from build123d import *

# Parameters (mm, degrees)
F0_W     = 127
F0_H     = 76.2
F1_DEPTH = 13.97
F3_D     = 12.7
F4_W     = 12.7
F4_H     = 25.4
F6_W     = 19.05
F6_H     = 12.372993
F8_W     = 9.582032
F8_H     = 12.456644
F10_R    = 2.54
F11_SIZE = 2.54
F12_SIZE = 2.54


with BuildPart() as f1:
    # F0 (on Top) → F1 (new body)
    with BuildSketch(Plane.XY):
        Rectangle(F0_W, F0_H)
    extrude(amount=F1_DEPTH)

    # F3 (through all)
    with Locations(Plane.XY.offset(13.97)):
        with Locations((-44.45, 26.67), (-44.45, -26.67), (44.45, 26.67), (44.45, -26.67)):
            Hole(F3_D / 2)

    # F4 (on Front) → F5 (revolve)
    with BuildSketch(Plane.XZ):
        with Locations((6.35, 26.67)):
            Rectangle(F4_W, F4_H)
    revolve(axis=Axis((0, 0, 26.67), (0, 0, -1)))

    # F6 (on Front) → F7 (revolve)
    with BuildSketch(Plane.XZ):
        with Locations((9.525, 45.556496)):
            Rectangle(F6_W, F6_H)
    revolve(axis=Axis((0, 0, 45.556497), (0, 0, -1)))

    # F8 (on Front) → F9 (revolve)
    with BuildSketch(Plane.XZ):
        with Locations((12.456648, 20.198322)):
            Rectangle(F8_W, F8_H)
    revolve(axis=Axis((0, 0, 13.97), (0, 0, 1)))

    # F10
    f10_edges = [f1.edges().sort_by_distance(p)[0] for p in [
        (-17.247664, 0, 26.426644),
        (-17.247664, 0, 13.97),
        (17.247664, 0, 20.198322),
    ]]
    fillet(f10_edges, radius=F10_R)

    # F11
    f11_edges = [f1.edges().sort_by_distance(p)[0] for p in [
        (-19.05, 0, 51.742993),
    ]]
    chamfer(f11_edges, length=F11_SIZE)

    # F12
    f12_edges = [f1.edges().sort_by_distance(p)[0] for p in [
        (0, -38.1, 13.97),
        (-63.5, 0, 13.97),
        (0, 38.1, 13.97),
        (63.5, 0, 13.97),
    ]]
    chamfer(f12_edges, length=F12_SIZE)


solid = f1.part
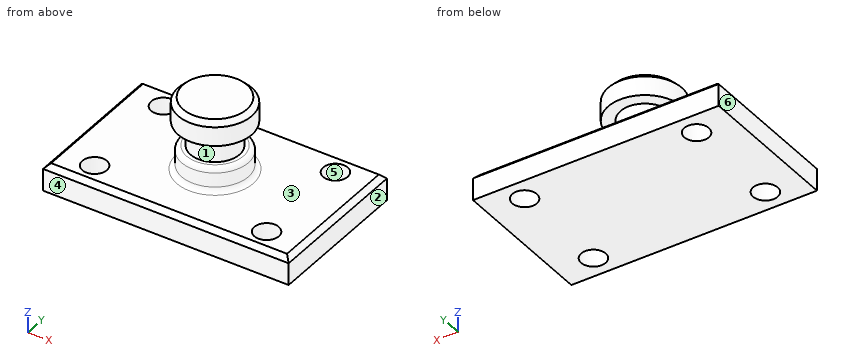
Model file for the job. Use its own axes, mm. Face numbers are marked on the shaded views. A direction names the side the tool comes from. Coordinates: 2 decimals unless noted, no trailing zeros. Write each loop counter-clockwise with the first axis right and the second up, starting at its lowest first coordinate (ties: lowest second). Pieces come first, ordered by that corner, then holes. Notation, with made-up numbers: (-32.5, 13.5) - (4.5, 13.5) arc R27 cw to (4.5, 35.5) - close; hole circle Ø3 at (31, 29). An arc over 180 degrees is marked (long way). Write each question's results on one line, items separated by ' | '. Start each with the question number.
1) 3-axis set-ups, long thin cutter, end or side, ignore diameter. For the marked faces 1, 2 and 3: which of +Z, -Z, +X, -X, +Y, -Y reach the whole face in a straight line?
2) Mould opens along Y. For the marked faces 4, 5 and 6 say: pulls with the +Y half, pulls with the -Y half, needs draft (parallel to the pull), parting line crosses it, or undercut.
3) Cut at C-C (x = 0). Write the cut outline in (y, z).
4) Cut at A-A (x = -44.45). Write the cut outline in (y, z), then the cut area to 3 significant figures.
5) Probe line 1 along Y through (x, z) = (-44.45, 6.5); line 2 along X through (y, z) = (26, 7); line 3 along X through (y, z) = (-21, 6). List the from-to ranges inside material, lowest first. Write a range as from..to.
6) Flat gauge pins, fed straight in: P1, Ø1.5, axis at x = -14.5, z = 15.5, coming from the +Y side; P2, Ø20.5, axis at x = -44.45, y = -26.67, coming from the +Z side; P3, Ø4, axis at x = -15, z = 46, coming from the -Y side. Where does each tip first touch, or does it go through?
7) Cut at D-D (z = 34). Write the cut outline in (x, y), then the cut area to 3 significant figures.
8) Cut at B-B (y = -26.67). Write the cut outline in (x, z).
Returned:
1) face 1: none | face 2: +Z, -Z, +X, +Y, -Y | face 3: +Z
2) face 4: pulls with the -Y half | face 5: undercut | face 6: needs draft
3) outline: (-38.1, 0) - (38.1, 0) - (38.1, 11.43) - (35.56, 13.97) - (19.79, 13.97) arc R2.54 cw to (17.25, 16.51) - (17.25, 23.89) arc R2.54 ccw to (14.71, 26.43) - (12.7, 26.43) - (12.7, 39.37) - (19.05, 39.37) - (19.05, 49.2) - (16.51, 51.74) - (-16.51, 51.74) - (-19.05, 49.2) - (-19.05, 39.37) - (-12.7, 39.37) - (-12.7, 26.43) - (-14.71, 26.43) arc R2.54 ccw to (-17.25, 23.89) - (-17.25, 16.51) arc R2.54 cw to (-19.79, 13.97) - (-35.56, 13.97) - (-38.1, 11.43) - close
4) outline: (-38.1, 0) - (-33.02, 0) - (-33.02, 13.97) - (-35.56, 13.97) - (-38.1, 11.43) - close; (-20.32, 0) - (20.32, 0) - (20.32, 13.97) - (-20.32, 13.97) - close; (33.02, 0) - (38.1, 0) - (38.1, 11.43) - (35.56, 13.97) - (33.02, 13.97) - close | area: 703 mm^2
5) line 1: -38.1..-33.02, -20.32..20.32, 33.02..38.1 | line 2: -63.5..-50.76, -38.14..38.14, 50.76..63.5 | line 3: -63.5..-47.31, -41.59..41.59, 47.31..63.5
6) P1: y = 10.98 | P2: z = 13.97 | P3: y = -13.92
7) outline: circle Ø25.4 at (0, 0) | area: 507 mm^2
8) outline: (-63.5, 0) - (-50.8, 0) - (-50.8, 13.97) - (-60.96, 13.97) - (-63.5, 11.43) - close; (-38.1, 0) - (38.1, 0) - (38.1, 13.97) - (-38.1, 13.97) - close; (50.8, 0) - (63.5, 0) - (63.5, 11.43) - (60.96, 13.97) - (50.8, 13.97) - close
